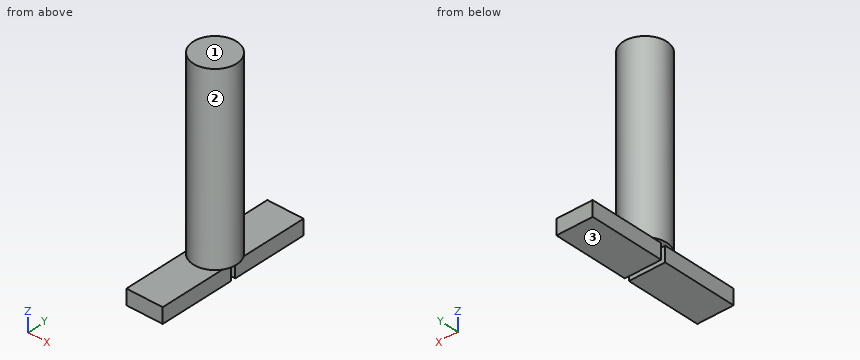
```python
from build123d import *

# Parameters (mm, degrees)
SKETCH1_R                = 7.13
BOSS_EXTRUDE1_DEPTH      = 60
BOSS_EXTRUDE2_DEPTH      = 0.01
BOSS_EXTRUDE2_DEPTH_BACK = 5
SKETCH2_W                = 12
SKETCH2_H                = 25


with BuildPart() as part:
    # Sketch1 → Boss-Extrude1 (new body)
    with BuildSketch(Plane.XY):
        Circle(SKETCH1_R)
    extrude(amount=BOSS_EXTRUDE1_DEPTH)

    # Sketch2 → Boss-Extrude2 (add, two sides: drawn at the far end of the back side and taken through both)
    with BuildSketch(Plane.XY.offset(-BOSS_EXTRUDE2_DEPTH_BACK)):
        with Locations((0, -13.25)):
            Rectangle(SKETCH2_W, SKETCH2_H)
        with Locations((0, 13.25)):
            Rectangle(SKETCH2_W, SKETCH2_H)
    extrude(amount=BOSS_EXTRUDE2_DEPTH + BOSS_EXTRUDE2_DEPTH_BACK)


solid = part.part
```
Build history of the part. All positions in model axes, mm. Face numbers are marked on the shaded views. Give positions to 0.01 mm unless a question says otherwise; leave off trailing zeros. Loops run counter-clockwise (first coordinate to the right, second up) from the corner with the lowest first, then second, coordinate; pieces in that order, holes last. Notation, with made-up numbers: (8, 67.5) -> (31, 67.5) arc R21 cw to (31, 95.5) -> close; hole circle Ø10 at (-4.5, 19). An arc over 180 degrees is marked (long way). One line per question, with ' | ' between items.
Q1. Drop flat-ended pins along their axis: pin 1 (1 mm diameter, centred on x = -5, z = 39.5, fed in from +Y); pin 2 (4 mm diameter, centred on y = 13, z = -1.5, fed in from -X); pin 3 (4 mm diameter, centred on y = -6, z = 43, fed in from -X); pin 4 (12 mm diameter, centred on y = -14, z = 11.5, fed in from -X). Give the stop position or say it passes through.
Filled sheet:
pin 1: stops at y = 5.53 | pin 2: stops at x = -6 | pin 3: stops at x = -5.9 | pin 4: passes through
Q2. Drill centre lines: line 1 along Y through (x, z) = (-5.25, -1); line 2 along Y through (x, z) = (-0.25, 26.5); line 3 along Z through (x, y) = (-0.5, 14.5). Where is each one in solid material? Low to high. Write a range as [from, to].
Filled sheet:
line 1: y = [-25.75, -0.75], [0.75, 25.75] | line 2: y = [-7.13, 7.13] | line 3: z = [-5, 0.01]
Q3. Cut at D-D, the plane x = 5.25. Write the cut outline in (y, z), plus the area to 3 significant figures.
Filled sheet:
outline: (-25.75, -5) -> (-0.75, -5) -> (-0.75, 0) -> (0.75, 0) -> (0.75, -5) -> (25.75, -5) -> (25.75, 0.01) -> (4.82, 0.01) -> (4.82, 60) -> (-4.82, 60) -> (-4.82, 0.01) -> (-25.75, 0.01) -> close | area: 829 mm²
Q4. Pull direction Z, two halves, no side cores. Call the marked faces 1, 2 and 3: pulls with the +Z half, pulls with the -Z half, needs draft (parallel to the pull), parting line crosses it, or undercut.
Filled sheet:
face 1: pulls with the +Z half | face 2: needs draft | face 3: pulls with the -Z half
Q5. Cut at A-A, the plane y = 6. Write the cut outline in (x, z), plus the area to 3 significant figures.
Filled sheet:
outline: (-6, -5) -> (6, -5) -> (6, 0.01) -> (3.85, 0.01) -> (3.85, 60) -> (-3.85, 60) -> (-3.85, 0.01) -> (-6, 0.01) -> close | area: 522 mm²
Q6. Cut at C-C, the plane z = 10.5. Write the cut outline in (x, y), plus the area to 3 significant figures.
Filled sheet:
outline: circle Ø14.26 at (0, 0) | area: 160 mm²
Q7. Cut at B-B, the plane x = 0. Write the cut outline in (y, z).
Filled sheet:
outline: (-25.75, -5) -> (-0.75, -5) -> (-0.75, 0) -> (0.75, 0) -> (0.75, -5) -> (25.75, -5) -> (25.75, 0.01) -> (7.13, 0.01) -> (7.13, 60) -> (-7.13, 60) -> (-7.13, 0.01) -> (-25.75, 0.01) -> close
